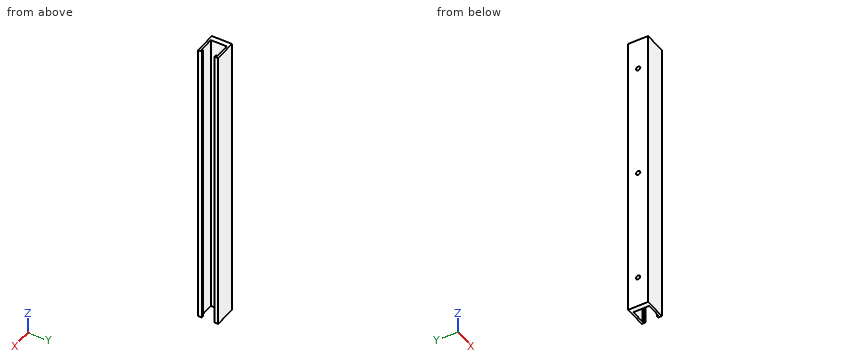
```python
from build123d import *

# Parameters (mm, degrees)
F0_W     = 21
F0_H     = 280
F1_DEPTH = 19
F3_DEPTH = 280.001
F4_R     = 2
F5_DEPTH = 4.8


with BuildPart() as f1:
    # F0 (on Front) → F1 (new body)
    with BuildSketch(Plane.XZ):
        with Locations((10.5, 140)):
            Rectangle(F0_W, F0_H)
    extrude(amount=F1_DEPTH)

    # F2 (on face) → F3 (cut, through all)
    with BuildSketch(Plane(origin=(0, 0, 0), x_dir=(1, 0, 0), z_dir=(0, 0, -1))):
        Polygon((19, 17), (4.8, 17), (4.8, 2), (19, 2), (19, 3.5), (21, 3.5), (21, 15.5), (19, 15.5), align=None)
    extrude(amount=-F3_DEPTH, mode=Mode.SUBTRACT)

    # F4 (on face) → F5 (cut, through all)
    with BuildSketch(Plane(origin=(0, 0, 0), x_dir=(0, -1, 0), z_dir=(-1, 0, 0))):
        with Locations((9.5, 30)):
            Circle(F4_R)
        with Locations((9.5, 140)):
            Circle(F4_R)
        with Locations((9.5, 250)):
            Circle(F4_R)
    extrude(amount=-F5_DEPTH, mode=Mode.SUBTRACT)


solid = f1.part
```
Read the model definition and answer for the solid it produces. Units are mm, in the model's axes. Round coordinates to 2 decimals unless told otherwise and drop trailing zeros. Write each loop counter-clockwise with the first axis right and the second up, starting at its lowest first coordinate (ties: lowest second). Pieces come first, ordered by that corner, then holes. Notation, with made-up numbers: (36.25, 25) - (67.25, 25) arc R16 cw to (67.25, 47) - close; hole circle Ø3 at (-15, 24.25). An arc over 180 degrees is marked (long way). One line per item, written item: value.
Q1. This flat-tipped pin is pushed along its axis until it touches: P1, Ø4, axis at y = -6, z = 206.5, coming from the +X side. Where does it stop, or does it pass through?
The answers:
P1: stops at x = 4.8
Q2. Straight lines are drawn through the part: line 1 (Z direction, x = 3.4, y = -9.5); line 2 (Y direction, x = 12.5, z = 108); line 3 (X direction, y = -16.75, z = 63). For each, find the intervals that lie inside material, in ascending order. Write a range as from..to.
The answers:
line 1: z = 0..28, 32..138, 142..248, 252..280
line 2: y = -19..-17, -2..0
line 3: x = 0..4.8, 19..21
Q3. Find section B-B (z = 182). Determine the outline of the cut face in (x, y).
The answers:
outline: (0, -19) - (21, -19) - (21, -15.5) - (19, -15.5) - (19, -17) - (4.8, -17) - (4.8, -2) - (19, -2) - (19, -3.5) - (21, -3.5) - (21, 0) - (0, 0) - close
Q4. Find section A-A (x = 11.25). Determine the outline of the cut face in (y, z), and give its area (3 significant figures).
The answers:
outline: (-19, 0) - (-17, 0) - (-17, 280) - (-19, 280) - close; (-2, 0) - (0, 0) - (0, 280) - (-2, 280) - close
area: 1,120 mm2
